```python
from build123d import *


with BuildPart() as part:
    # Schizzo1 → Rivoluzione1 (revolve)
    with BuildSketch(Plane.XY):
        with BuildLine():
            Line((-0.5, 51.75), (0.5, 51.75))
            ThreePointArc((0.5, 51.75), (1.207106781, 51.457106781), (1.5, 50.75))
            Line((1.5, 50.75), (1.5, 49.75))
            ThreePointArc((1.5, 49.75), (1.207106781, 49.042893219), (0.5, 48.75))
            Line((0.5, 48.75), (-0.5, 48.75))
            ThreePointArc((-0.5, 48.75), (-1.207106781, 49.042893219), (-1.5, 49.75))
            Line((-1.5, 49.75), (-1.5, 50.75))
            ThreePointArc((-1.5, 50.75), (-1.207106781, 51.457106781), (-0.5, 51.75))
        make_face()
    revolve(axis=Axis((0, 0, 0), (1, 0, 0)))


solid = part.part
```
Read the model definition and answer for the solid it produces. Units are mm, in the model's axes. Give positions to 0.01 mm unless a question says otherwise; leave off trailing zeros. Write each loop counter-clockwise with the first axis right and the second up, starting at its lowest first coordinate (ties: lowest second). Pieces come first, ordered by that corner, then holes. Notation, with made-up numbers: (-19.5, 77) -> (13.5, 77) arc R26 cw to (13.5, 113) -> close; hole circle Ø9 at (46, 58.25). An arc over 180 degrees is marked (long way). Answer in a Markdown table with one row per item.
1) Section A-A on z = 0 is taken. Give the vertices of the cut face in (x, y).
Results list:
| item | result |
|---|---|
| outline | (-1.5, -50.75) arc R1 ccw to (-0.5, -51.75) -> (0.5, -51.75) arc R1 ccw to (1.5, -50.75) -> (1.5, -49.75) arc R1 ccw to (0.5, -48.75) -> (-0.5, -48.75) arc R1 ccw to (-1.5, -49.75) -> close; (-1.5, 49.75) arc R1 ccw to (-0.5, 48.75) -> (0.5, 48.75) arc R1 ccw to (1.5, 49.75) -> (1.5, 50.75) arc R1 ccw to (0.5, 51.75) -> (-0.5, 51.75) arc R1 ccw to (-1.5, 50.75) -> close |
2) Straight lines are drawn through the part: line 1 (Z direction, x = 0.25, y = 0); line 2 (Y direction, x = 1.2, z = 38); line 3 (Y direction, x = -1, z = -28). For each, find the intervals that lie inside material, in ascending order. Write a range as [from, to].
Results list:
| item | result |
|---|---|
| line 1 | [-51.75, -48.75], [48.75, 51.75] |
| line 2 | [-34.71, -30.99], [30.99, 34.71] |
| line 3 | [-43.36, -40.07], [40.07, 43.36] |
3) Determine the mould class of faces 1 (the cylindrical face through (-0.01, -38.69, -29.66)), 2 (the flat face through (1.5, 34, -37)), 3 (the cylindrical face through (0.01, 49.36, 15.54)) for opening direction Z: released by +Z, released by -Z, zero draft, split by the parting line, or undercut.
Results list:
| item | result |
|---|---|
| face 1 | undercut |
| face 2 | zero draft |
| face 3 | split by the parting line |
